Part print with two shaded views. Sizes in mm from the minimum x, y, z corner. A direction names the side the tool comes from. Round coordinates to 2 decimals unless told otherwise and drop trailing zeros. Write each loop counter-clockwise with the first axis right and the second up, starting at its lowest first coordinate (ties: lowest second). Pieces come first, ordered by that corner, then holes. Notation, with made-up numbers: (87, 68.5) -> (96, 68.5) arc R24 cw to (96, 83.5) -> close; hole circle Ø10 at (18.25, -0.5). An arc over 180 degrees is marked (long way). Return JSON: item names as keys, results as strings.
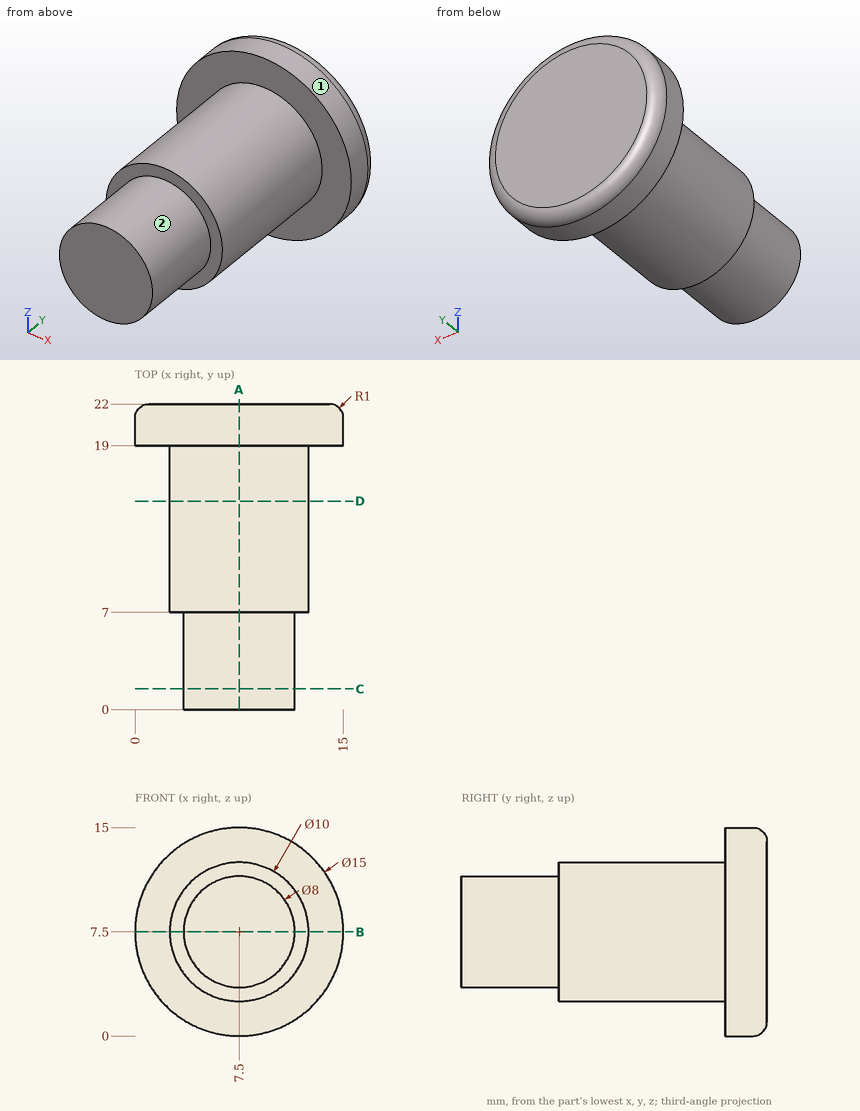
Q1. Saw through at A-A on x = 7.5. List the corners of the cut face in (y, z).
Verdict:
{"outline": "(0, 3.5) -> (7, 3.5) -> (7, 2.5) -> (19, 2.5) -> (19, 0) -> (21, 0) arc R1 ccw to (22, 1) -> (22, 14) arc R1 ccw to (21, 15) -> (19, 15) -> (19, 12.5) -> (7, 12.5) -> (7, 11.5) -> (0, 11.5) -> close"}
Q2. Saw through at D-D on y = 15. List the corners of the cut face in (x, z), then the cut area to 3 significant figures.
Verdict:
{"outline": "circle Ø10 at (7.5, 7.5)", "area": "78.5 mm²"}
Q3. Saw through at B-B on z = 7.5. List the corners of the cut face in (x, y).
Verdict:
{"outline": "(0, 19) -> (2.5, 19) -> (2.5, 7) -> (3.5, 7) -> (3.5, 0) -> (11.5, 0) -> (11.5, 7) -> (12.5, 7) -> (12.5, 19) -> (15, 19) -> (15, 21) arc R1 ccw to (14, 22) -> (1, 22) arc R1 ccw to (0, 21) -> close"}
Q4. Wall check: L1, parallel to Y at x = 4, z = 10.25; L2, parallel to Y at x = 4.5, z = 2.5; L3, parallel to X at y = 20.25, z = 11. Give the ranges that are in metal, low to high.
Verdict:
{"L1": "y = 7 to 22", "L2": "y = 19 to 22", "L3": "x = 0.87 to 14.13"}
Q5. 3-axis set-ups, long thin cutter, end or side, ignore diameter. For the marked faces 1 and 2: which of +Z, -Z, +X, -X, +Y, -Y reach the whole face in a straight line?
Verdict:
{"face 1": "+Y, -Y", "face 2": "-Y"}
Q6. Saw through at C-C on y = 1.5. List the corners of the cut face in (x, z).
Verdict:
{"outline": "circle Ø8 at (7.5, 7.5)"}
Q7. Pin check, flat tips, straight feed: pin 1 Ø5 at (y, z) = (8, 2) entering from -X; pin 2 Ø1 at (y, z) = (19.5, 10.5) entering from +X; pin 3 Ø4 at (y, z) = (12, 9) entering from -X. Stop position of each tip, or through.
Verdict:
{"pin 1": "stops at x = 3.5", "pin 2": "stops at x = 14.57", "pin 3": "stops at x = 2.5"}
